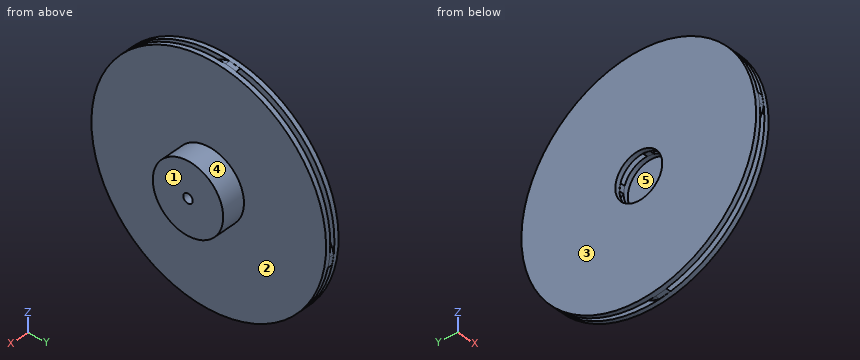
from build123d import *

# Parameters (mm, degrees)
BOSS_EXTRUDE1_DEPTH   = 1
BOSS_EXTRUDE1_2_DEPTH = 1
BOSS_EXTRUDE1_3_DEPTH = 1
BOSS_EXTRUDE1_4_DEPTH = 1
SKETCH2_R             = 25
SKETCH2_R_2           = 5
BOSS_EXTRUDE2_DEPTH   = 1
BOSS_EXTRUDE6_START   = -1
SKETCH2_4_R           = 25
SKETCH2_4_R_2         = 5
BOSS_EXTRUDE6_DEPTH   = 1
SKETCH3_R             = 7.5
BOSS_EXTRUDE7_DEPTH   = 5
SKETCH4_R             = 1
CUT_EXTRUDE1_DEPTH    = 4


with BuildPart() as part:
    # Sketch1 → Boss-Extrude1 (new body)
    with BuildSketch(Plane(origin=(0, 0, 0), x_dir=(0, 0, -1), z_dir=(1, 0, 0))):
        with BuildLine():
            add(Edge.make_bspline(
                [(0, 5), (4.497529661, 10.734535644), (18.077265621, 8.404390401), (22.903151971, -1.371454076), (24.494897428, -5)],
                knots=[0, 0, 0, 0, 0.618777628, 1, 1, 1, 1], degree=3))
            add(Edge.make_bspline(
                [(24.494897428, -5), (24.856687291, -2.673031407)],
                knots=[0, 0, 1, 1], degree=1))
            add(Edge.make_bspline(
                [(-1.492986361, 4.77189603), (-1.334435901, 6.923416971), (1.516351493, 9.375782971), (6.922460383, 11.063211687), (12.668210337, 10.322852941), (18.630485351, 7.165584221), (22.391904574, 2.350944019), (24.550618301, -1.104983558), (24.856687291, -2.673031407)],
                knots=[0, 0, 0, 0, 0.172506063, 0.296264897, 0.482616547, 0.652804407, 0.864378799, 1, 1, 1, 1], degree=3))
            add(Edge.make_bspline(
                [(-1.492986361, 4.77189603), (0, 5)],
                knots=[0, 0, 1, 1], degree=1))
        make_face()
    extrude(amount=BOSS_EXTRUDE1_DEPTH)



with BuildPart() as body_2:
    # Sketch1 → Boss-Extrude1 2 (new body)
    with BuildSketch(Plane(origin=(0, 0, 0), x_dir=(0, 0, -1), z_dir=(1, 0, 0))):
        with BuildLine():
            add(Edge.make_bspline(
                [(4.77189603, 1.492986361), (6.923416971, 1.334435901), (9.375782971, -1.516351493), (11.063211687, -6.922460383), (10.322852941, -12.668210337), (7.165584221, -18.630485351), (2.350944019, -22.391904574), (-1.104983558, -24.550618301), (-2.673031407, -24.856687291)],
                knots=[0, 0, 0, 0, 0.172506063, 0.296264897, 0.482616547, 0.652804407, 0.864378799, 1, 1, 1, 1], degree=3))
            add(Edge.make_bspline(
                [(-5, -24.494897428), (-2.673031407, -24.856687291)],
                knots=[0, 0, 1, 1], degree=1))
            add(Edge.make_bspline(
                [(5, 0), (10.734535644, -4.497529661), (8.404390401, -18.077265621), (-1.371454076, -22.903151971), (-5, -24.494897428)],
                knots=[0, 0, 0, 0, 0.618777628, 1, 1, 1, 1], degree=3))
            add(Edge.make_bspline(
                [(4.77189603, 1.492986361), (5, 0)],
                knots=[0, 0, 1, 1], degree=1))
        make_face()
    extrude(amount=BOSS_EXTRUDE1_2_DEPTH)


with BuildPart() as body_3:
    # Sketch1 → Boss-Extrude1 3 (new body)
    with BuildSketch(Plane(origin=(0, 0, 0), x_dir=(0, 0, -1), z_dir=(1, 0, 0))):
        with BuildLine():
            add(Edge.make_bspline(
                [(1.492986361, -4.77189603), (1.334435901, -6.923416971), (-1.516351493, -9.375782971), (-6.922460383, -11.063211687), (-12.668210337, -10.322852941), (-18.630485351, -7.165584221), (-22.391904574, -2.350944019), (-24.550618301, 1.104983558), (-24.856687291, 2.673031407)],
                knots=[0, 0, 0, 0, 0.172506063, 0.296264897, 0.482616547, 0.652804407, 0.864378799, 1, 1, 1, 1], degree=3))
            add(Edge.make_bspline(
                [(-24.494897428, 5), (-24.856687291, 2.673031407)],
                knots=[0, 0, 1, 1], degree=1))
            add(Edge.make_bspline(
                [(0, -5), (-4.497529661, -10.734535644), (-18.077265621, -8.404390401), (-22.903151971, 1.371454076), (-24.494897428, 5)],
                knots=[0, 0, 0, 0, 0.618777628, 1, 1, 1, 1], degree=3))
            add(Edge.make_bspline(
                [(1.492986361, -4.77189603), (0, -5)],
                knots=[0, 0, 1, 1], degree=1))
        make_face()
    extrude(amount=BOSS_EXTRUDE1_3_DEPTH)


with BuildPart() as body_4:
    # Sketch1 → Boss-Extrude1 4 (new body)
    with BuildSketch(Plane(origin=(0, 0, 0), x_dir=(0, 0, -1), z_dir=(1, 0, 0))):
        with BuildLine():
            add(Edge.make_bspline(
                [(-4.77189603, -1.492986361), (-6.923416971, -1.334435901), (-9.375782971, 1.516351493), (-11.063211687, 6.922460383), (-10.322852941, 12.668210337), (-7.165584221, 18.630485351), (-2.350944019, 22.391904574), (1.104983558, 24.550618301), (2.673031407, 24.856687291)],
                knots=[0, 0, 0, 0, 0.172506063, 0.296264897, 0.482616547, 0.652804407, 0.864378799, 1, 1, 1, 1], degree=3))
            add(Edge.make_bspline(
                [(5, 24.494897428), (2.673031407, 24.856687291)],
                knots=[0, 0, 1, 1], degree=1))
            add(Edge.make_bspline(
                [(-5, 0), (-10.734535644, 4.497529661), (-8.404390401, 18.077265621), (1.371454076, 22.903151971), (5, 24.494897428)],
                knots=[0, 0, 0, 0, 0.618777628, 1, 1, 1, 1], degree=3))
            add(Edge.make_bspline(
                [(-4.77189603, -1.492986361), (-5, 0)],
                knots=[0, 0, 1, 1], degree=1))
        make_face()
    extrude(amount=BOSS_EXTRUDE1_4_DEPTH)


with BuildPart() as part_1:
    add(part.part)

    add(body_2.part)  # Boss-Extrude2 merges body 2

    add(body_3.part)  # Boss-Extrude2 merges body 3

    add(body_4.part)  # Boss-Extrude2 merges body 4
    # Sketch2 → Boss-Extrude2 (add)
    with BuildSketch(Plane(origin=(1, 0, 0), x_dir=(0, 0, -1), z_dir=(1, 0, 0))):
        Circle(SKETCH2_R)
        Circle(SKETCH2_R_2, mode=Mode.SUBTRACT)
    extrude(amount=BOSS_EXTRUDE2_DEPTH)

    # Sketch2<4> → Boss-Extrude6 (add)
    with BuildSketch(Plane(origin=(1, 0, 0), x_dir=(0, 0, -1), z_dir=(1, 0, 0)).offset(BOSS_EXTRUDE6_START)):
        Circle(SKETCH2_4_R)
        Circle(SKETCH2_4_R_2, mode=Mode.SUBTRACT)
    extrude(amount=-BOSS_EXTRUDE6_DEPTH)

    # Sketch3 → Boss-Extrude7 (add)
    with BuildSketch(Plane(origin=(2, 0, 0), x_dir=(0, 0, -1), z_dir=(1, 0, 0))):
        Circle(SKETCH3_R)
    extrude(amount=BOSS_EXTRUDE7_DEPTH)

    # Sketch4 → Cut-Extrude1 (cut)
    with BuildSketch(Plane(origin=(7, 0, 0), x_dir=(0, 0, -1), z_dir=(1, 0, 0))):
        Circle(SKETCH4_R)
    extrude(amount=-CUT_EXTRUDE1_DEPTH, mode=Mode.SUBTRACT)


solid = part_1.part
Geometry check sheet. Reference: the model listing, model coordinates, mm. Face numbers are marked on the shaded views. A direction names the side the tool comes from. Coordinates: 2 decimals unless noted, no trailing zeros. Order: outer loops, then holes, each group sorted by start corner. A loop starts at its lowest first (then second) coordinate and runs counter-clockwise, first axis right, second up. Notation, with made-up numbers: M 12.25,5 L 56.25,5 A21 ccw 56.25,27 Z; hole C 31.5,6.25 d4. An arc over 180 degrees is marked long. Use CSV: the item, a comma, the result in double quotes.
Item 1: Mould release check, pull along Z, two halves, no side actions. Record for the marked faces 3, 4 and 5: pulls with the +Z half, pulls with the -Z half, needs draft (parallel to the pull), parting line crosses it, or undercut.
Returned:
face 3,"needs draft"
face 4,"parting line crosses it"
face 5,"undercut"
Item 2: Tool access check on the marked faces 1 and 2. Record the directions out of +Z, -Z, +X, -X, +Y, -Y that give a thin tool (end or side, any length) a straight path to the whole face; none if there is none.
Returned:
face 1,"+Z, -Z, +X, +Y, -Y"
face 2,"+X"
Item 3: Cross-section at A-A on x = 5.25. Record the cut outline in (y, z), then the cut area to 3 significant figures.
Returned:
outline,"C 0,0 d15; hole C 0,0 d2"
area,"174 mm2"
Item 4: Cross-section at B-B on z = -6.5. Give the number of separate pieces and of enclosed holes in the cut face, then the cut area to 3 significant figures.
Returned:
separate pieces,"1"
enclosed holes,"2"
area,"141 mm2"
Item 5: Gauge pin test, flat ends, axial feed: pin 1 Ø1 at (y, z) = (10.5, -18.5) entering from +X; pin 2 Ø13.5 at (y, z) = (0, -8) entering from +X; pin 3 Ø4 at (x, y) = (3.5, -7.5) entering from +Z; pin 4 Ø1.6 at (y, z) = (0, 0) entering from +X. Record the tip position at first contact, or that the pin passes through.
Returned:
pin 1,"stops at x = 2"
pin 2,"stops at x = 7"
pin 3,"stops at z = 24.22"
pin 4,"stops at x = 3"
Item 6: Thickness scan on line 1 along Y through (x, z) = (-0.65, 0); line 2 along X through (y, z) = (-18, 2); line 3 along Y through (x, z) = (4.7, 0). Record the ranges inside material, lowest first.
Returned:
line 1,"y = -25 to -5, 5 to 25"
line 2,"x = -1 to 0, 1 to 2"
line 3,"y = -7.5 to -1, 1 to 7.5"
